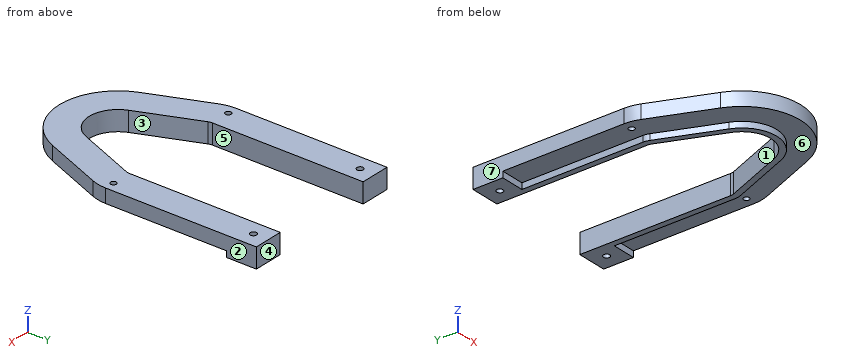
Autodesk Inventor part; units mm, degrees
ref_plane "YZ Plane" through (0, 0, 0) normal (1, 0, 0) x (0, 1, 0)
ref_plane "XZ Plane" through (0, 0, 0) normal (0, 1, 0) x (-1, 0, 0)
ref_plane "XY Plane" through (0, 0, 0) normal (0, 0, 1) x (1, 0, 0)
sketch "Sketch13" plane through (0, 0, 0) normal (0, 0, 1) x (1, 0, 0)
  line L0 (-247.6922, -121.6988) -> (-240.7003, -114.707)
  line L1 (-240.7003, -114.707) -> (-206.5582, -114.707)
  line L2 (-206.5582, -114.707) -> (-199.5663, -121.6988)
  line L3 (-199.5663, -121.6988) -> (-199.5663, -165.5825)
  arc A0 (-199.7872, -166.7122) -> (-199.5663, -165.5825) centre (-202.5663, -165.5825) ccw
  line L4 (-199.7872, -166.7122) -> (-212.0494, -196.8785)
  arc A1 (-235.2091, -196.8785) -> (-212.0494, -196.8785) centre (-223.6293, -192.1714) ccw
  line L5 (-235.2091, -196.8785) -> (-247.4714, -166.7122)
  arc A2 (-247.6922, -165.5825) -> (-247.4714, -166.7122) centre (-244.6922, -165.5825) ccw
  line L6 (-247.6922, -165.5825) -> (-247.6922, -121.6988)
  circle A3 centre (-223.6293, -151.1714) radius 13
  line L7 (26.8154, -89.707) -> (-473.1846, -89.707)
  line L8 (26.8154, -104.707) -> (-473.1846, -104.707)
  line L9 (-197.5663, -165.5825) -> (-197.5663, -120.8704)
  line L10 (-197.5663, -120.8704) -> (-205.7298, -112.707)
  line L11 (-205.7298, -112.707) -> (-241.5288, -112.707)
  line L12 (-241.5288, -112.707) -> (-249.6922, -120.8704)
  line L13 (-249.6922, -120.8704) -> (-249.6922, -165.5825)
  arc A4 (-249.6922, -165.5825) -> (-249.3242, -167.4653) centre (-244.6922, -165.5825) ccw
  line L14 (-249.3242, -167.4653) -> (-237.0619, -197.6316)
  arc A5 (-237.0619, -197.6316) -> (-210.1966, -197.6316) centre (-223.6293, -192.1714) ccw
  line L15 (-210.1966, -197.6316) -> (-197.9344, -167.4653)
  arc A6 (-197.9344, -167.4653) -> (-197.5663, -165.5825) centre (-202.5663, -165.5825) ccw
  line L16 (-182.5663, -165.5825) -> (-182.5663, -114.6572)
  line L17 (-182.5663, -114.6572) -> (-199.5166, -97.707)
  line L18 (-199.5166, -97.707) -> (-247.742, -97.707)
  line L19 (-247.742, -97.707) -> (-264.6922, -114.6572)
  line L20 (-264.6922, -114.6572) -> (-264.6922, -165.5825)
  arc A7 (-264.6922, -165.5825) -> (-263.22, -173.1138) centre (-244.6922, -165.5825) ccw
  line L21 (-263.22, -173.1138) -> (-250.9578, -203.2801)
  arc A8 (-250.9578, -203.2801) -> (-196.3008, -203.2801) centre (-223.6293, -192.1714) ccw
  line L22 (-196.3008, -203.2801) -> (-184.0385, -173.1138)
  arc A9 (-184.0385, -173.1138) -> (-182.5663, -165.5825) centre (-202.5663, -165.5825) ccw
  line L23 (-182.5663, -114.6572) -> (-182.5663, -89.707)
  line L24 (-264.6922, -114.6572) -> (-264.6922, -89.707)
  line L25 (-197.5663, -120.8704) -> (-197.5663, -89.707)
  line L26 (-249.6922, -120.8704) -> (-249.6922, -89.707)
  line L27 (-218.4828, -188.996) -> (-218.1293, -188.6424)
  line L28 (-218.1293, -188.6424) -> (-218.1293, -184.996)
  line L29 (-218.1293, -184.996) -> (-229.1293, -184.996)
  line L30 (-229.1293, -184.996) -> (-229.1293, -188.6424)
  line L31 (-229.1293, -188.6424) -> (-228.7757, -188.996)
  line L32 (-228.9525, -189.3022) -> (-229.4355, -189.1728)
  line L33 (-229.4355, -189.1728) -> (-232.5934, -190.996)
  line L34 (-223.806, -198.2161) -> (-228.9525, -189.3022)
  line L35 (-227.0934, -200.5223) -> (-223.9355, -198.6991)
  line L36 (-223.9355, -198.6991) -> (-223.806, -198.2161)
  line L37 (-223.4525, -198.2161) -> (-223.3231, -198.6991)
  line L38 (-223.3231, -198.6991) -> (-220.1652, -200.5223)
  line L39 (-218.306, -189.3022) -> (-223.4525, -198.2161)
  line L40 (-214.6652, -190.996) -> (-217.8231, -189.1728)
  line L41 (-217.8231, -189.1728) -> (-218.306, -189.3022)
  line L42 (-228.7757, -188.996) -> (-218.4828, -188.996)
  line L43 (-232.5934, -190.996) -> (-227.0934, -200.5223)
  line L44 (-220.1652, -200.5223) -> (-214.6652, -190.996)
  point P0 (0, 0)
  dimension "d26" = 2
  dimension "d27" = 15
extrude "Extrusion14" add sketch "Sketch13" along normal blind 10 contours L23 L8 L17 L25 L7 | L23 L17 L8 | L26 L19 L8 L24 L7 | L17 L8 L25 | L17 L16 A9 L22 A8 L21 A7 L20 L19 L8 L26 L13 A4 L14 A5 L15 A6 L9 L25 | L26 L8 L19 | L8 L19 L24
sketch "Sketch14" plane through (0, 0, 0) normal (0, 0, -1) x (-1, 0, 0)
  line L0 (249.6922, -165.5825) -> (249.6922, -89.707)
  arc A0 (249.3242, -167.4653) -> (249.6922, -165.5825) centre (244.6922, -165.5825) ccw
  line L1 (237.0619, -197.6316) -> (249.3242, -167.4653)
  arc A1 (210.1966, -197.6316) -> (237.0619, -197.6316) centre (223.6293, -192.1714) ccw
  line L2 (197.9344, -167.4653) -> (210.1966, -197.6316)
  arc A2 (197.5663, -165.5825) -> (197.9344, -167.4653) centre (202.5663, -165.5825) ccw
  line L3 (197.5663, -89.707) -> (197.5663, -165.5825)
  line L4 (182.5663, -89.707) -> (197.5663, -89.707)
  line L5 (182.5663, -165.5825) -> (182.5663, -89.707)
  arc A3 (182.5663, -165.5825) -> (184.0385, -173.1138) centre (202.5663, -165.5825) ccw
  line L6 (196.3008, -203.2801) -> (184.0385, -173.1138)
  arc A4 (196.3008, -203.2801) -> (250.9578, -203.2801) centre (223.6293, -192.1714) ccw
  line L7 (263.22, -173.1138) -> (250.9578, -203.2801)
  arc A5 (263.22, -173.1138) -> (264.6922, -165.5825) centre (244.6922, -165.5825) ccw
  line L8 (264.6922, -89.707) -> (264.6922, -165.5825)
  line L9 (249.6922, -89.707) -> (264.6922, -89.707)
  line L10 (185.5663, -92.707) -> (194.5663, -92.707)
  line L11 (194.5663, -92.707) -> (194.5663, -165.5825)
  arc A6 (194.5663, -165.5825) -> (195.1552, -168.595) centre (202.5663, -165.5825) ccw
  line L12 (195.1552, -168.595) -> (207.4175, -198.7613)
  arc A7 (207.4175, -198.7613) -> (239.8411, -198.7613) centre (223.6293, -192.1714) ccw
  line L13 (239.8411, -198.7613) -> (252.1033, -168.595)
  arc A8 (252.1033, -168.595) -> (252.6922, -165.5825) centre (244.6922, -165.5825) ccw
  line L14 (252.6922, -165.5825) -> (252.6922, -92.707)
  line L15 (252.6922, -92.707) -> (261.6922, -92.707)
  line L16 (261.6922, -92.707) -> (261.6922, -165.5825)
  arc A9 (260.4408, -171.9841) -> (261.6922, -165.5825) centre (244.6922, -165.5825) ccw
  line L17 (260.4408, -171.9841) -> (248.1786, -202.1504)
  arc A10 (199.0799, -202.1504) -> (248.1786, -202.1504) centre (223.6293, -192.1714) ccw
  line L18 (199.0799, -202.1504) -> (186.8177, -171.9841)
  arc A11 (185.5663, -165.5825) -> (186.8177, -171.9841) centre (202.5663, -165.5825) ccw
  line L19 (185.5663, -165.5825) -> (185.5663, -92.707)
  line L20 (194.5663, -92.707) -> (194.5663, -89.707)
  line L21 (182.5663, -89.707) -> (197.5663, -89.707)
  line L22 (252.6922, -92.707) -> (252.6922, -89.707)
  line L23 (197.5663, -89.707) -> (197.5663, -165.5825)
  line L24 (197.5663, -104.707) -> (182.5663, -104.707)
  line L25 (264.6922, -89.707) -> (264.6922, -165.5825)
  line L26 (264.6922, -104.707) -> (249.6922, -104.707)
  point P0 (0, 0)
  point P1 (194.5663, -104.707)
  point P2 (264.6922, -104.707)
  point P3 (252.6922, -104.707)
  dimension "d33" = 3
  dimension "d34" = 15
extrude "Extrusion15" cut sketch "Sketch14" against normal blind 3 contours L26 L16 A9 L17 A10 L18 A11 L19 L24 L11 A6 L12 A7 L13 A8 L14 | L26 L8 A5 L7 A4 L6 A3 L5 L24 L19 A11 L18 A10 L17 A9 L16
sketch "Sketch15" plane through (0, 0, 3) normal (0, 0, -1) x (-1, 0, 0)
  line L0 (182.5663, -165.5825) -> (182.5663, -104.707)
  line L1 (264.6922, -104.707) -> (264.6922, -165.5825)
  point P0 (0, 0)
  point P1 (187.5663, -165.5825)
  point P2 (259.6922, -165.5825)
  dimension "d35" = 5
  dimension "d36" = 5
hole "Hole1" at (-187.5663, -165.5825, 3) at (-259.6922, -165.5825, 3) direction (0, 0, 1) diameter 2.9 end through all
sketch "Sketch16" plane through (0, 0, 10) normal (0, 0, 1) x (1, 0, 0)
  line L0 (-264.6922, -89.707) -> (-264.6922, -165.5825)
  line L1 (-182.5663, -165.5825) -> (-182.5663, -89.707)
  point P0 (0, 0)
  point P1 (-257.1922, -97.207)
  point P2 (-190.0663, -97.207)
  dimension "d44" = 7.5
  dimension "d45" = 7.5
  dimension "d46" = 7.5
hole "Hole2" at (-257.1922, -97.207, 10) at (-190.0663, -97.207, 10) direction (0, 0, -1) diameter 3.2 end through all
properties part number "Rear Cover Bracket" material "ABS Plastic"
Could you check a few things on this model? Use its own coordinates, in mm. Face numbers are marked on the shaded views. A direction names the side the tool comes from. Round coordinates to 2 decimals unless told otherwise and drop trailing zeros. Write each loop counter-clockwise with the first axis right and the second up, starting at its lowest first coordinate (ties: lowest second). Pieces come first, ordered by that corner, then holes. Notation, with made-up numbers: M -30.75,47 L -8.75,47 A9 cw -8.75,58 Z; hole C 79.5,16 d11. An arc over 180 degrees is marked long. Write each question's results on one line, items separated by ' | '. Start each with the question number.
1. On a 3-axis mill with a long thin cutter (end or side, diameter ignored), from which of +Z, -Z, +X, -X, +Y, -Y can I reach the whole of each face in a straight line? I mean the marked faces 5, 6 and 7. Say none if no direction works.
2. Imagine slicing it at D-D on x = -244.5. List the corners of the cut face in (y, z) for me, and give its area (3 significant figures).
3. Imagine slicing it at C-C on y = -211. List the corners of the cut face in (x, z) for me.
4. Thinking about a two-plate mould opening in X: for the marked faces 1, 2, 3 and 4, which applies, +X half, -X half, draft (parallel to the pull), parting line (faces both ways), or undercut?
5. Imagine slicing it at B-B on x = -227.5. List the corners of the cut face in (y, z) for me.
6. Imagine slicing it at A-A on y = -161.5. List the corners of the cut face in (x, z) for me, and give its area (3 significant figures).
7. I need wall thicknesses on L1, parallel to X at y = -114, z = 4; L2, parallel to X at y = -107.5, z = 0.5; L3, parallel to X at y = -166.5, z = 6.5 (1 decimal). Which ranges of each line are inside material? Lowest first, please. Write a range as from..to.
8. I'm going to push flat-ended pins straight in: pin 1 Ø2.5 at (x, z) = (-187, 1.5) entering from -Y; pin 2 Ø3 at (x, z) = (-213, 2) entering from -Y; pin 3 Ø1 at (x, z) = (-233, 5) entering from +Y. Where does each tip first touch, or does it pass through?
Result sheet:
1) face 5: +Z, -Z, +Y | face 6: -Z, -Y | face 7: +Z, -Z, -X, +Y, -Y
2) outline: M -213.02,3 L -187.3,3 L -187.3,0 L -179.33,0 L -179.33,10 L -213.02,10 Z | area: 260 mm^2
3) outline: M -246.34,3 L -200.92,3 L -200.92,10 L -246.34,10 Z
4) face 1: undercut | face 2: +X half | face 3: undercut | face 4: draft
5) outline: M -221.42,3 L -209.24,3 L -209.24,0 L -206.15,0 L -206.15,10 L -221.42,10 Z
6) outline: M -264.69,3 L -252.69,3 L -252.69,0 L -249.69,0 L -249.69,10 L -264.69,10 Z; M -197.57,0 L -194.57,0 L -194.57,3 L -182.57,3 L -182.57,10 L -197.57,10 Z | area: 228 mm^2
7) L1: x = -264.69..-249.69, -197.57..-182.57 | L2: x = -252.69..-249.69, -197.57..-194.57 | L3: x = -264.7..-260.8, -258.6..-249.6, -197.7..-188.7, -186.4..-182.6
8) pin 1: stops at y = -104.71 | pin 2: stops at y = -220.1 | pin 3: stops at y = -202.79
